The listing builds one solid part. Answer for the finished solid, in the listing's coordinates (mm). Coordinates: 2 decimals unless noted, no trailing zeros. Order: outer loops, then holes, each group sorted by start corner. A loop starts at its lowest first (then second) coordinate and runs counter-clockwise, first axis right, second up. Notation, with made-up numbers: (11, -20.75) - (29, -20.75) arc R16 cw to (29, 4.25) - close; hole circle Ø4 at (36.5, -36). An arc over 180 degrees is marked (long way). Use one line per item in the form item = value. Start each with the question number.
Item 1: This flat-tipped pin is pushed along its axis until it touches: pin 1 Ø2 at (x, z) = (2, -4.5) entering from -Y. Where does it stop, or does it pass through?
Item 2: Consider line 1 along X through (y, z) = (0.65, 0); line 2 along Z through (x, y) = (3, 0.45); line 3 along Z through (x, y) = (6.5, 0.25). Determine where each line is inside the solid, lowest interval first. Write a range as [from, to].
Item 3: Section D-D, the plane z = -7.25 is taken. Write down the section's boundary in (x, y), and give its area (3 significant figures).
Item 4: Section A-A, the plane x = 0 is taken. Write down the section's boundary in (y, z), and give its area (3 significant figures).
Item 5: Section C-C, the plane y = 0.15 is taken. Write down the section's boundary in (x, z).
Item 6: Section B-B, the plane z = 0 is taken. Write down the section's boundary in (x, y).
from build123d import *

# Parameters (mm, degrees)
BOSS_EXTRUDE1_DEPTH = 0.8
FILLET1_R           = 0.1


with BuildPart() as part:
    # Sketch1 → Boss-Extrude1 (new body)
    with BuildSketch(Plane(origin=(0, 0, 0), x_dir=(1, 0, 0), z_dir=(0, 1, 0))):
        with BuildLine():
            ThreePointArc((9.786805864, 3.803739078), (3.026060815, 10.054499288), (-6.061654374, 8.573584213))
            ThreePointArc((-6.061654374, 8.573584213), (-7.260490637, 8.07091926), (-8.559417578, 8.122583993))
            ThreePointArc((-8.559417578, 8.122583993), (-3.400715964, -11.299342057), (11.620731486, 2.049048496))
            ThreePointArc((11.620731486, 2.049048496), (10.509059049, 2.722891827), (9.786805864, 3.803739078))
        make_face()
        with BuildLine():
            Line((-1.5, 6.5), (1.5, 6.5))
            Line((1.5, 6.5), (1.5, 7.858116823))
            ThreePointArc((1.5, 7.858116823), (0, -8), (-1.5, 7.858116823))
            Line((-1.5, 7.858116823), (-1.5, 6.5))
        make_face(mode=Mode.SUBTRACT)
    extrude(amount=BOSS_EXTRUDE1_DEPTH)

    # Fillet1
    fillet1_edges = [part.edges().sort_by_distance(p)[0] for p in [
        (-1.5, 0.4, -7.858116823),
        (1.5, 0.4, -7.858116823),
    ]]
    fillet(fillet1_edges, radius=FILLET1_R)


solid = part.part
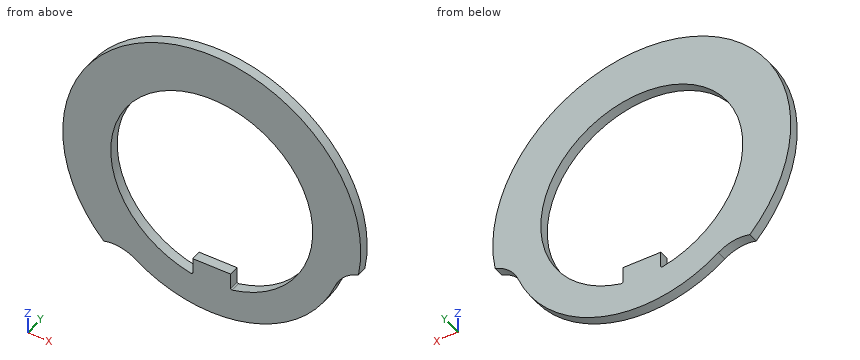
Response:
q1.pin_1 = through
q2.line_1 = [-11.8, -8], [8, 11.8]
q2.line_2 = [-10.06, -7.42], [7.42, 11.41]
q2.line_3 = [-8.25, -4.66], [4.66, 9.85]
q3.outline = (-9.31, 0) - (-3.38, 0) - (-3.38, 0.8) - (-9.31, 0.8) - close; (-1.5, 0) - (1.5, 0) - (1.5, 0.8) - (-1.5, 0.8) - close; (3.38, 0) - (7.6, 0) - (7.6, 0.8) - (3.38, 0.8) - close
q3.area = 10.5 mm2
q4.outline = (0, -10.5) - (0.8, -10.5) - (0.8, -6.5) - (0, -6.5) - close; (0, 8) - (0.8, 8) - (0.8, 11.8) - (0, 11.8) - close
q4.area = 6.24 mm2
q5.outline = (-8.56, -8.12) arc R3 cw to (-6.06, -8.57) arc R10.5 ccw to (9.79, -3.8) arc R3 cw to (11.62, -2.05) arc R11.8 ccw (long way) to start; hole (-1.62, -7.83) arc R0.1 ccw to (-1.5, -7.74) - (-1.5, -6.5) - (1.5, -6.5) - (1.5, -7.74) arc R0.1 ccw to (1.62, -7.83) arc R8 ccw (long way) to start
q6.outline = (-11.8, 0) - (-8, 0) - (-8, 0.8) - (-11.8, 0.8) - close; (8, 0) - (11.8, 0) - (11.8, 0.8) - (8, 0.8) - close
